Read the model definition and answer for the solid it produces. Units are mm, in the model's axes. Give positions to 0.01 mm unless a question says otherwise; leave off trailing zeros. Order: outer loops, then holes, each group sorted by start corner. A loop starts at its lowest first (then second) coordinate and runs counter-clockwise, first axis right, second up.
Item 1: A cutting plane is placed at B-B (y = 15). Write down the section's boundary in (x, z).
Item 2: Find the intervals of material crossed by line 1 along Y through (x, z) = (20, 7); line 2 along Y through (x, z) = (201.4, 2.5); line 3 along X through (y, z) = (9.5, 6), in increasing order.
Item 3: A cutting plane is placed at D-D (x = 20). Write down the section's boundary in (y, z).
Item 4: A cutting plane is placed at C-C (z = 8.5). Write down the section's boundary in (x, y).
Item 5: A cutting plane is placed at A-A (x = 201.4). Write down the section's boundary in (y, z).
Item 6: The mould has two halves that part along X. Classify faces 1 (the face through (199, 13.2, 6.1)), 2 (the face through (221.4, 15, 6)), 3 (the face through (112, 30, 6)): +X half, -X half, draft (parallel to the pull), parting line (faces both ways), or undercut.
Autodesk Inventor part; units mm, degrees
ref_plane "YZ Plane" through (0, 0, 0) normal (1, 0, 0) x (0, 1, 0)
ref_plane "XZ Plane" through (0, 0, 0) normal (0, 1, 0) x (-1, 0, 0)
ref_plane "XY Plane" through (0, 0, 0) normal (0, 0, 1) x (1, 0, 0)
sketch "Sketch1" plane through (0, 0, 0) normal (0, 0, 1) x (1, 0, 0)
  line L0 (0, 0) -> (221.4, 0)
  line L1 (221.4, 0) -> (221.4, 30)
  line L2 (221.4, 30) -> (0, 30)
  line L3 (0, 30) -> (0, 0)
  dimension "d0" = 221.4
  dimension "d1" = 30
extrude "Extrusion1" add sketch "Sketch1" along normal blind 12
fillet "Fillet1" radius 5 4 edges at (221.4, 30, 6) (221.4, 0, 6) (0, 0, 6) (0, 30, 6)
sketch "Sketch2" plane through (0, 0, 12) normal (0, 0, 1) x (1, 0, 0)
  line L0 (0, 25) -> (0, 5)
  line L1 (0, 15) -> (20, 15)
  circle A0 centre (20, 15) radius 6
  line L2 (5, 0) -> (216.4, 0)
  line L3 (110.7, 0) -> (110.7, 30)
  line L4 (216.4, 30) -> (5, 30)
  line L5 (221.4, 5) -> (221.4, 25)
  line L6 (221.4, 15) -> (201.4, 15)
  circle A1 centre (201.4, 15) radius 3
  point P0 (0, 0)
  dimension "d5" = 20
  dimension "d6" = 12
  dimension "d10" = 20
  dimension "d11" = 6
extrude "Extrusion2" cut sketch "Sketch2" against normal through all
ref_plane "Work Plane1" through (0, 0, 6) normal (0, 0, 1) x (1, 0, 0)
properties part number "Fourbar-Crank"
Response values:
1. outline: (0, 0) - (14, 0) - (14, 12) - (0, 12) - close; (26, 0) - (198.4, 0) - (198.4, 12) - (26, 12) - close; (204.4, 0) - (221.4, 0) - (221.4, 12) - (204.4, 12) - close
2. line 1: y = 0 to 9, 21 to 30
2. line 2: y = 0 to 12, 18 to 30
2. line 3: x = 0 to 17.6, 22.4 to 221.4
3. outline: (0, 0) - (9, 0) - (9, 12) - (0, 12) - close; (21, 0) - (30, 0) - (30, 12) - (21, 12) - close
4. outline: (0, 5) arc R5 ccw to (5, 0) - (216.4, 0) arc R5 ccw to (221.4, 5) - (221.4, 25) arc R5 ccw to (216.4, 30) - (5, 30) arc R5 ccw to (0, 25) - close; hole circle Ø12 at (20, 15); hole circle Ø6 at (201.4, 15)
5. outline: (0, 0) - (12, 0) - (12, 12) - (0, 12) - close; (18, 0) - (30, 0) - (30, 12) - (18, 12) - close
6. face 1: undercut
6. face 2: +X half
6. face 3: draft
